The model under review builds one solid part; all positions refer to its coordinate system, in mm. Coordinates: 2 decimals unless noted, no trailing zeros. Order: outer loops, then holes, each group sorted by start corner. A loop starts at its lowest first (then second) coordinate and runs counter-clockwise, first axis right, second up. Notation, with made-up numbers: (-14.75, -37) -> (40.25, -37) arc R21 cw to (40.25, -19) -> close; hole circle Ø10 at (-2.75, 10.5). An arc over 180 degrees is marked (long way). Put each result on its own line as item: value.
from build123d import *

# Parameters (mm, degrees)
SZKIC1_W = 3
SZKIC1_H = 5
SZKIC2_W = 157
SZKIC2_H = 2.5


with BuildPart() as part:
    # Szkic1 → Obr_t1 (revolve)
    with BuildSketch(Plane(origin=(0, 0, 0), x_dir=(0, 0, -1), z_dir=(1, 0, 0)), mode=Mode.PRIVATE) as obr_t1_sk:
        with Locations((-1.5, 2.5)):
            Rectangle(SZKIC1_W, SZKIC1_H)
    revolve(obr_t1_sk.sketch.rotate(Axis((0, 0, 0), (0, 0, 1)), 270), axis=Axis((0, 0, 0), (0, 0, 1)))

    # Szkic2 → Obr_t2 (revolve)
    with BuildSketch(Plane(origin=(0, 0, 0), x_dir=(0, 0, -1), z_dir=(1, 0, 0)), mode=Mode.PRIVATE) as obr_t2_sk:
        with Locations((-81.5, 1.25)):
            Rectangle(SZKIC2_W, SZKIC2_H)
    revolve(obr_t2_sk.sketch.rotate(Axis((0, 0, 3), (0, 0, 1)), 270), axis=Axis((0, 0, 3), (0, 0, 1)))

    # Szkic3 → Obr_t3 (revolve)
    with BuildSketch(Plane(origin=(0, 0, 0), x_dir=(0, 0, -1), z_dir=(1, 0, 0)), mode=Mode.PRIVATE) as obr_t3_sk:
        with BuildLine():
            Line((-3.3, 2.5), (-3, 2.5))
            Line((-3, 2.5), (-3, 2.8))
            ThreePointArc((-3, 2.8), (-3.087867966, 2.587867966), (-3.3, 2.5))
        make_face()
    revolve(obr_t3_sk.sketch.rotate(Axis((0, 0, 0), (0, 0, 1)), 270), axis=Axis((0, 0, 0), (0, 0, 1)))


solid = part.part
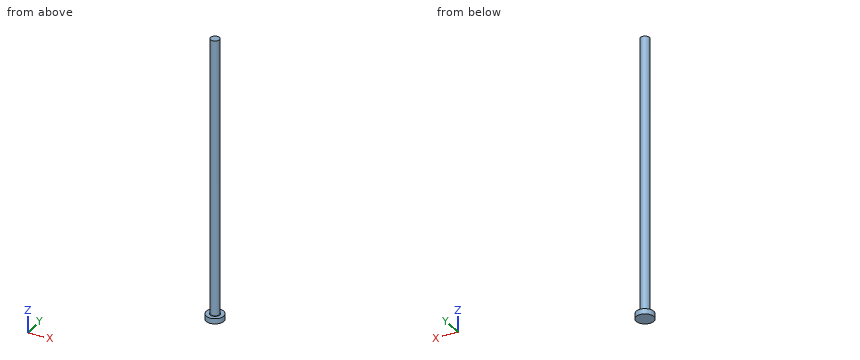
Item 1: Consider section C-C on z = 49.5. Write out the cut boundary in (x, y).
Answers below:
outline: circle Ø5 at (0, 0)
Item 2: For line 1 (Z direction, x = 1.5, y = -3.75); line 2 (Y direction, x = -1, z = 143.5); line 3 (Y direction, x = -0.5, z = 19), list the stretches that pass through material, from the lowest coordinate up. Write a range as from..to.
Answers below:
line 1: 0..3
line 2: -2.29..2.29
line 3: -2.45..2.45
Item 3: For pin 1 Ø1.5 at (y, z) = (0.5, 37) entering from -X; pin 2 Ø1.5 at (x, y) = (-3.5, -4) entering from +Z; pin 3 Ø1.5 at (x, y) = (2.5, 0.5) entering from +Z; pin 4 Ø2 at (x, z) = (-3, 128) entering from -Y, all flat-tipped, find the tip position at first contact; note any pin that passes through.
Answers below:
pin 1: x = -2.5
pin 2: z = 3
pin 3: z = 160
pin 4: y = -1.5
Item 4: Consider section A-A on y = 0. Write out the cut boundary in (x, z).
Answers below:
outline: (-5, 0) -> (5, 0) -> (5, 3) -> (2.8, 3) arc R0.3 cw to (2.5, 3.3) -> (2.5, 160) -> (-2.5, 160) -> (-2.5, 3.3) arc R0.3 cw to (-2.8, 3) -> (-5, 3) -> close
